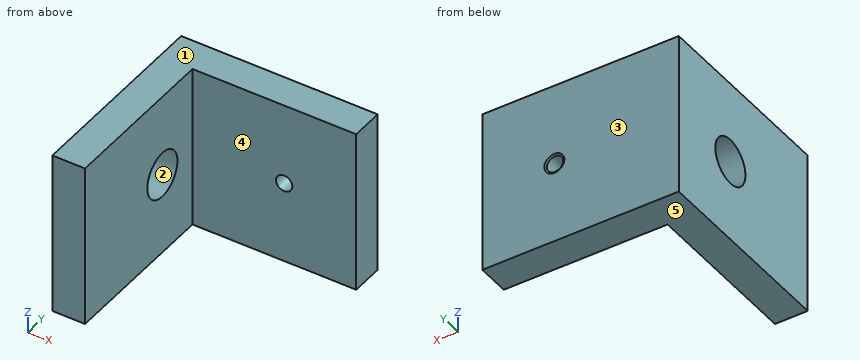
```python
from build123d import *

# Parameters (mm, degrees)
ESTRUSIONE_ESTRUSIONE1_DEPTH    = 25
SCHIZZO2_R                      = 3.5
TAGLIO_ESTRUSIONE1_DEPTH        = 25
FORO_FILETTATO_M3_1_D           = 2.5
FORO_FILETTATO_M3_1_DEPTH       = 8.5
FORO_FILETTATO_M3_1_CSINK_D     = 3.05
FORO_FILETTATO_M3_1_CSINK_ANGLE = 120
FORO_FILETTATO_M3_1_TIP         = 0.751075774


with BuildPart() as part:
    # Schizzo1 → Estrusione-Estrusione1 (new body)
    with BuildSketch(Plane.XY):
        Polygon((0, 0), (0, 30), (30, 30), (30, 25), (5, 25), (5, 0), align=None)
    extrude(amount=ESTRUSIONE_ESTRUSIONE1_DEPTH)

    # Schizzo2 → Taglio-Estrusione1 (cut)
    with BuildSketch(Plane.ZY):
        with Locations((12.5, 18)):
            Circle(SCHIZZO2_R)
    extrude(amount=-TAGLIO_ESTRUSIONE1_DEPTH, mode=Mode.SUBTRACT)

    # Foro filettato M3-1
    with Locations(Plane(origin=(0, 30, 0), x_dir=(1, 0, 0), z_dir=(0, 1, 0))):
        with Locations((19, -12.5)):
            CounterSinkHole(FORO_FILETTATO_M3_1_D / 2, FORO_FILETTATO_M3_1_CSINK_D / 2, depth=FORO_FILETTATO_M3_1_DEPTH, counter_sink_angle=FORO_FILETTATO_M3_1_CSINK_ANGLE)
            with Locations((0, 0, -(FORO_FILETTATO_M3_1_DEPTH + FORO_FILETTATO_M3_1_TIP / 2))):  # 118° drill point
                Cone(0, FORO_FILETTATO_M3_1_D / 2, FORO_FILETTATO_M3_1_TIP, mode=Mode.SUBTRACT)


solid = part.part
```
The listing builds one solid part. Answer for the finished solid, in the listing's coordinates (mm). Face numbers are marked on the shaded views. A direction names the side the tool comes from. Coordinates: 2 decimals unless noted, no trailing zeros. Loops run counter-clockwise (first coordinate to the right, second up) from the corner with the lowest first, then second, coordinate; pieces in that order, holes last. Notation, with made-up numbers: M 50.5,21 L 103.5,21 A14 cw 103.5,39 Z; hole C 84,-32.5 d6. An arc over 180 degrees is marked long. Answer as CSV lines item,"result". Start each with the question number.
(1) The part is cut by section A-A (x = 19). Give the vertices of the cut face in (y, z) (3 decimals), and give its area (3 significant figures).
(2) Given pin 1 (2 mm diameter, centred on x = 25.5, y = 23, fed in from +Z); pin 2 (7.5 mm diameter, centred on x = 16, z = 12, fed in from -Y); pin 3 (9 mm diameter, centred on y = 18, z = 12.5, fed in from +X), each flat-ended and moving along its own axis, determine where each tip first touches the part or whether it passes through.
(3) Find the intervals of material crossed by L1, parallel to Y at x = 3, z = 12.5; L2, parallel to Y at x = 21.75, z = 23.25; L3, parallel to X at y = 7.25, z = 6.75, in increasing order. Write a range as [from, to].
(4) The part is cut by section C-C (z = 12.5). Give the vertices of the cut face in (x, y) (3 decimals).
(5) The part is cut by section B-B (y = 18). Give the vertices of the cut face in (x, z).
(6) For the marked faces 4 and 5, determine the directions among +Z, -Z, +X, -X, +Y, -Y from which every point of the face is accessible in a straight line to the end or side of a thin tool.
(7) The mould has two halves that part along Z. Classify the marked faces 1, 2 and 3: pulls with the +Z half, pulls with the -Z half, needs draft (parallel to the pull), parting line crosses it, or undercut.
(8) The part is cut by section D-D (x = 2). Give the vertices of the cut face in (y, z).
Determined:
1,outline,"M 25,0 L 30,0 L 30,10.975 L 29.841,11.25 L 25,11.25 Z; M 25,13.75 L 29.841,13.75 L 30,14.025 L 30,25 L 25,25 Z"
1,area,"112 mm2"
2,pin 1,"through"
2,pin 2,"y = 25"
2,pin 3,"x = 5"
3,L1,"[0, 14.5], [21.5, 30]"
3,L2,"[25, 30]"
3,L3,"[0, 5]"
4,outline,"M 0,0 L 5,0 L 5,14.5 L 0,14.5 Z; M 0,21.5 L 5,21.5 L 5,25 L 17.75,25 L 17.75,29.841 L 17.475,30 L 0,30 Z; M 20.25,25 L 30,25 L 30,30 L 20.525,30 L 20.25,29.841 Z"
5,outline,"M 0,0 L 5,0 L 5,9 L 0,9 Z; M 0,16 L 5,16 L 5,25 L 0,25 Z"
6,face 4,"+Z, -Z, +X, -Y"
6,face 5,"-Z, +X, -X, +Y, -Y"
7,face 1,"pulls with the +Z half"
7,face 2,"undercut"
7,face 3,"needs draft"
8,outline,"M 0,0 L 30,0 L 30,25 L 0,25 Z; hole C 18,12.5 d7"
